Geometry: see drawing. Coordinates: mm, zero at the bounding-box minimum. A direction names the side the tool comes from. Give positions to 0.01 mm unless a question says otherwise; leave off trailing zeros. Write each loop counter-clockwise with the first axis right and the second up, starting at its lowest first coordinate (ties: lowest second). Pieces come first, ordered by that corner, then holes. Notation, with made-up numbers: M 14,-29 L 61,-29 A27 cw 61,-9 Z; hole C 29,34.5 d9. An arc over 180 degrees is marked long. Use one line per item in the form item = value. Start each with the question number.
Item 1: Section query A-A on x = 3.3. Return loops of the section in (y, z), then the cut area to 3 significant figures.
Item 2: Contact query for flat-ended pins moving along their axis: P1, Ø1, axis at x = 11, z = 8.5, coming from the +Y side; P2, Ø2.5, axis at y = 31.5, z = 14.5, coming from the -X side; P3, Ø2, axis at x = 4.5, z = 7, coming from the -Y side. Output: stop coordinate, or through.
Item 3: Access query for the marked faces 1, 2, 3 and 4. Directions: +Z, -Z, +X, -X, +Y, -Y. A direction counts if a zero-diameter tool reaches every point of the face in a straight line with its end or side. Return the directions, or none.
Item 4: Section query C-C on z = 6.5. Return loops of the section in (x, y), then the cut area to 3 significant figures.
Item 5: Material intervals for line 1 along Z through (x, y) = (3.3, 27.4); line 2 along X through (y, z) = (27.65, 16.3); line 3 along Y through (x, z) = (47, 12), sorted ascending. Write a range as from..to.
Item 6: Section query B-B on z = 3.7. Return loops of the section in (x, y), then the cut area to 3 significant figures.
Item 7: Section query D-D on x = 35. Return loops of the section in (y, z).
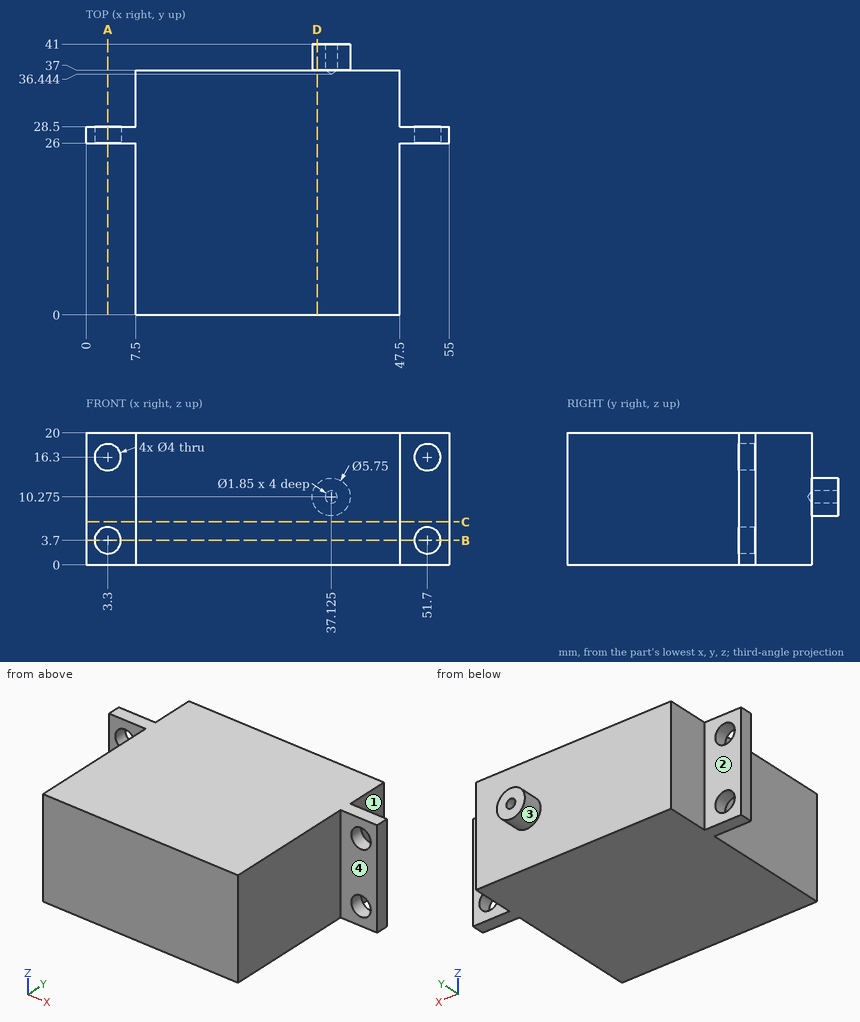
Answer sheet:
q1.outline = M 26,0 L 28.5,0 L 28.5,1.7 L 26,1.7 Z; M 26,5.7 L 28.5,5.7 L 28.5,14.3 L 26,14.3 Z; M 26,18.3 L 28.5,18.3 L 28.5,20 L 26,20 Z
q1.area = 30.0 mm2
q2.P1 = 37
q2.P2 = 7.5
q2.P3 = 26
q3.face_1 = +Z, -Z, +X, +Y
q3.face_2 = +Z, -Z, -X, +Y
q3.face_3 = +Y
q3.face_4 = +Z, -Z, +X, -Y
q4.outline = M 0,26 L 7.5,26 L 7.5,0 L 47.5,0 L 47.5,26 L 55,26 L 55,28.5 L 47.5,28.5 L 47.5,37 L 7.5,37 L 7.5,28.5 L 0,28.5 Z
q4.area = 1,520 mm2
q5.line_1 = 0..1.7, 5.7..14.3, 18.3..20
q5.line_2 = 0..1.3, 5.3..49.7, 53.7..55
q5.line_3 = 0..37
q6.outline = M 0,26 L 1.3,26 L 1.3,28.5 L 0,28.5 Z; M 5.3,26 L 7.5,26 L 7.5,0 L 47.5,0 L 47.5,26 L 49.7,26 L 49.7,28.5 L 47.5,28.5 L 47.5,37 L 7.5,37 L 7.5,28.5 L 5.3,28.5 Z; M 53.7,26 L 55,26 L 55,28.5 L 53.7,28.5 Z
q6.area = 1,500 mm2
q7.outline = M 0,0 L 37,0 L 37,8.34 L 41,8.34 L 41,12.21 L 37,12.21 L 37,20 L 0,20 Z
